from build123d import *

# Parameters (mm, degrees)
SKETCH2_R           = 2.159
BOSS_EXTRUDE3_DEPTH = 3.81
SKETCH1_R           = 38.5318
SKETCH1_R_2         = 35.9918
CUT_EXTRUDE1_DEPTH  = 0.4445
SKETCH4_R           = 25.781
CUT_EXTRUDE2_DEPTH  = 3.81
BOSS_EXTRUDE4_DEPTH = 12.7
BOSS_EXTRUDE5_DEPTH = 6.35
CUT_EXTRUDE3_START  = -3.81
CUT_EXTRUDE3_DEPTH  = 3.81
BOSS_EXTRUDE6_DEPTH = 15.875
CUT_EXTRUDE4_REACH  = 72.276
SKETCH12_R          = 4.2164


with BuildPart() as part:
    # Sketch2 → Boss-Extrude3 (new body)
    with BuildSketch(Plane(origin=(0, 0, 0), x_dir=(1, 0, 0), z_dir=(0, 1, 0))):
        with BuildLine():
            Line((34.29, 46.99), (-34.29, 46.99))
            ThreePointArc((-34.29, 46.99), (-43.270256121, 43.270256121), (-46.99, 34.29))
            Line((-46.99, 34.29), (-46.99, -34.29))
            ThreePointArc((-46.99, -34.29), (-43.270256121, -43.270256121), (-34.29, -46.99))
            Line((-34.29, -46.99), (34.29, -46.99))
            ThreePointArc((34.29, -46.99), (43.270256121, -43.270256121), (46.99, -34.29))
            Line((46.99, -34.29), (46.99, 34.29))
            ThreePointArc((46.99, 34.29), (43.270256121, 43.270256121), (34.29, 46.99))
        make_face()
        with Locations(Location((0, 41.275, 0), (0, 0, 270))):
            Circle(SKETCH2_R, mode=Mode.SUBTRACT)
        with Locations(Location((29.185832393, 29.185832393, 0), (0, 0, 270))):
            Circle(SKETCH2_R, mode=Mode.SUBTRACT)
        with Locations(Location((41.275, 0, 0), (0, 0, 270))):
            Circle(SKETCH2_R, mode=Mode.SUBTRACT)
        with Locations(Location((29.185832393, -29.185832393, 0), (0, 0, 270))):
            Circle(SKETCH2_R, mode=Mode.SUBTRACT)
        with Locations(Location((0, -41.275, 0), (0, 0, 270))):
            Circle(SKETCH2_R, mode=Mode.SUBTRACT)
        with Locations(Location((-29.185832393, -29.185832393, 0), (0, 0, 270))):
            Circle(SKETCH2_R, mode=Mode.SUBTRACT)
        with Locations(Location((-41.275, 0, 0), (0, 0, 270))):
            Circle(SKETCH2_R, mode=Mode.SUBTRACT)
        with Locations(Location((-29.185832393, 29.185832393, 0), (0, 0, 270))):
            Circle(SKETCH2_R, mode=Mode.SUBTRACT)
    extrude(amount=-BOSS_EXTRUDE3_DEPTH)

    # Sketch1 → Cut-Extrude1 (cut)
    with BuildSketch(Plane(origin=(0, 0, 0), x_dir=(1, 0, 0), z_dir=(0, 1, 0))):
        with Locations(Location((0, 0, 0), (0, 0, 270))):
            Circle(SKETCH1_R)
        with Locations(Location((0, 0, 0), (0, 0, 270))):
            Circle(SKETCH1_R_2, mode=Mode.SUBTRACT)
    extrude(amount=-CUT_EXTRUDE1_DEPTH, mode=Mode.SUBTRACT)

    # Sketch4 → Cut-Extrude2 (cut)
    with BuildSketch(Plane(origin=(0, 0, 0), x_dir=(1, 0, 0), z_dir=(0, 1, 0))):
        with Locations(Location((0, 0, 0), (0, 0, 270))):
            Circle(SKETCH4_R)
    extrude(amount=-CUT_EXTRUDE2_DEPTH, mode=Mode.SUBTRACT)

    # Sketch5 → Boss-Extrude4 (add)
    with BuildSketch(Plane.XZ.offset(3.81)):
        with BuildLine():
            ThreePointArc((-29.083, 16.035), (-25.261329281, 25.261329281), (-16.035, 29.083))
            Line((-16.035, 29.083), (16.035, 29.083))
            ThreePointArc((16.035, 29.083), (25.261329281, 25.261329281), (29.083, 16.035))
            Line((29.083, 16.035), (29.083, -16.035))
            ThreePointArc((29.083, -16.035), (25.261329281, -25.261329281), (16.035, -29.083))
            Line((16.035, -29.083), (-16.035, -29.083))
            ThreePointArc((-16.035, -29.083), (-25.261329281, -25.261329281), (-29.083, -16.035))
            Line((-29.083, -16.035), (-29.083, 16.035))
        make_face()
        with BuildLine():
            Line((-26.035, -16.035), (-26.035, 16.035))
            ThreePointArc((-26.035, 16.035), (-23.106067812, 23.106067812), (-16.035, 26.035))
            Line((-16.035, 26.035), (16.035, 26.035))
            ThreePointArc((16.035, 26.035), (23.106067812, 23.106067812), (26.035, 16.035))
            Line((26.035, 16.035), (26.035, -16.035))
            ThreePointArc((26.035, -16.035), (23.106067812, -23.106067812), (16.035, -26.035))
            Line((16.035, -26.035), (-16.035, -26.035))
            ThreePointArc((-16.035, -26.035), (-23.106067812, -23.106067812), (-26.035, -16.035))
        make_face(mode=Mode.SUBTRACT)
    extrude(amount=BOSS_EXTRUDE4_DEPTH)

    # Sketch6 → Boss-Extrude5 (add)
    with BuildSketch(Plane.XZ.offset(16.51)):
        with BuildLine():
            Line((-29.083, 16.035), (-29.083, -16.035))
            ThreePointArc((-29.083, -16.035), (-25.261329281, -25.261329281), (-16.035, -29.083))
            Line((-16.035, -29.083), (16.035, -29.083))
            ThreePointArc((16.035, -29.083), (25.261329281, -25.261329281), (29.083, -16.035))
            Line((29.083, -16.035), (29.083, 16.035))
            ThreePointArc((29.083, 16.035), (25.261329281, 25.261329281), (16.035, 29.083))
            Line((16.035, 29.083), (-16.035, 29.083))
            ThreePointArc((-16.035, 29.083), (-25.261329281, 25.261329281), (-29.083, 16.035))
        make_face()
    extrude(amount=BOSS_EXTRUDE5_DEPTH)

    # Sketch7 → Cut-Extrude3 (cut)
    with BuildSketch(Plane.XZ.offset(3.81).offset(CUT_EXTRUDE3_START)):
        with BuildLine():
            Line((-46.99, 34.29), (-46.99, 0))
            ThreePointArc((-46.99, 0), (-33.226947648, 33.226947648), (0, 46.99))
            Line((0, 46.99), (-34.29, 46.99))
            ThreePointArc((-34.29, 46.99), (-43.270256121, 43.270256121), (-46.99, 34.29))
        make_face()
        with BuildLine():
            ThreePointArc((0, -46.99), (-33.226947648, -33.226947648), (-46.99, 0))
            Line((-46.99, 0), (-46.99, -34.29))
            ThreePointArc((-46.99, -34.29), (-43.270256121, -43.270256121), (-34.29, -46.99))
            Line((-34.29, -46.99), (0, -46.99))
        make_face()
    extrude(amount=CUT_EXTRUDE3_DEPTH, mode=Mode.SUBTRACT)

    # Sketch8 → Boss-Extrude6 (add, symmetric)
    with BuildSketch(Plane(origin=(0, 0, 0), x_dir=(0, 0, -1), z_dir=(1, 0, 0))):
        Polygon((-29.083, -3.81), (-29.083, -11.43), (-34.163, -3.81), align=None)
    boss_extrude6 = extrude(amount=BOSS_EXTRUDE6_DEPTH, both=True)

    # Mirror1: Boss-Extrude6 across plane
    add(boss_extrude6.mirror(Plane.XY))

    # Sketch12 → Cut-Extrude4 (cut, up to next)
    with BuildSketch(Plane.XZ.offset(22.86), mode=Mode.PRIVATE) as cut_extrude4_sk1:
        with Locations(Location((-16.035, 16.035, 0), (0, 0, 270))):
            Circle(SKETCH12_R)
    cut_extrude4_tool1 = extrude(cut_extrude4_sk1.sketch, amount=-CUT_EXTRUDE4_REACH, mode=Mode.PRIVATE) & part.part
    # Sketch12 → Cut-Extrude4 (cut, up to next)
    with BuildSketch(Plane.XZ.offset(22.86), mode=Mode.PRIVATE) as cut_extrude4_sk2:
        with Locations(Location((16.035, -16.035, 0), (0, 0, 270))):
            Circle(SKETCH12_R)
    cut_extrude4_tool2 = extrude(cut_extrude4_sk2.sketch, amount=-CUT_EXTRUDE4_REACH, mode=Mode.PRIVATE) & part.part
    # Sketch12 → Cut-Extrude4 (cut, up to next)
    with BuildSketch(Plane.XZ.offset(22.86), mode=Mode.PRIVATE) as cut_extrude4_sk3:
        with Locations(Location((0, 0, 0), (0, 0, 270))):
            Circle(SKETCH12_R)
    cut_extrude4_tool3 = extrude(cut_extrude4_sk3.sketch, amount=-CUT_EXTRUDE4_REACH, mode=Mode.PRIVATE) & part.part
    add(cut_extrude4_tool1.solids().sort_by_distance((-16.035, -22.86, 16.035))[0], mode=Mode.SUBTRACT)
    add(cut_extrude4_tool2.solids().sort_by_distance((16.035, -22.86, -16.035))[0], mode=Mode.SUBTRACT)
    add(cut_extrude4_tool3.solids().sort_by_distance((0, -22.86, 0))[0], mode=Mode.SUBTRACT)


solid = part.part
Design review of the part built by this model. Coordinates are the model's own, in mm. A direction names the side the tool comes from. Give positions to 0.01 mm unless a question says otherwise; leave off trailing zeros. Order: outer loops, then holes, each group sorted by start corner. A loop starts at its lowest first (then second) coordinate and runs counter-clockwise, first axis right, second up. Notation, with made-up numbers: (30, 29) - (82, 29) arc R26 cw to (82, 65) - close; hole circle Ø1 at (4.5, 46). An arc over 180 degrees is marked (long way). Use CSV: the item, a comma, the result in double quotes. Start each with the question number.
Q1. Take a section at B-B (y = -8.5). State the section outline as (x, z) points (3 decimals).
Q2. For line 1 (X direction, y = -1, z = 0); line 2 (X direction, y = -0.15, z = 0); line 3 (X direction, y = -21.25, z = 0), list the stretches that pass through material, from the lowest coordinate up.
Q3. Draft analysis for pull direction Y (two halves, no side actions). For faces 4 (the face through (0, -22.86, 7)), 5 (the face through (23.18, -10.07, -23.03)), 6 (the face through (43.416, -1.878, -0.281)), 7 (the face through (-23.18, -10.07, 23.03)), state which applies: pulls with the +Y half, pulls with the -Y half, needs draft (parallel to the pull), parting line crosses it, or undercut.
Q4. Take a section at D-D (z = -24). State the section outline as (x, y) points, and give its area (3 significant figures).
Q5. For P1, Ø10, axis at x = 5, y = -16, coming from the -Z side; P2, Ø10, axis at x = -4.5, y = -12, coming from the +Z side; P3, Ø5.5, axis at x = 1, y = -15.5, coming from the -Z side, all flat-tipped, find the tip position at first contact; note any pin that passes through.
Q6. Take a section at A-A (y = -20.5). State the section outline as (x, z) points (3 decimals), and give its area (3 significant figures).
Q7. Take a section at C-C (y = -2.25). Count the separate pieces of the cut face and the enclosed holes in it, and give its area (3 significant figures).
Q8. Machinability: for faces 1 (the face through (25.16, -13.2, -25.36)), 2 (the face through (-15.875, -7, -31)), 3 (the face through (15.875, -7, 31)), which of the approach directions +Z, -Z, +X, -X, +Y, -Y give a long, thin tool a straight path to every point of the face, cutting with its end or side? Answer none if there is none.
Calculated:
1,outline,"(-29.083, -16.035) arc R13.048 ccw to (-16.035, -29.083) - (-15.875, -29.083) - (-15.875, -31.036) - (15.875, -31.036) - (15.875, -29.083) - (16.035, -29.083) arc R13.048 ccw to (29.083, -16.035) - (29.083, 16.035) arc R13.048 ccw to (16.035, 29.083) - (15.875, 29.083) - (15.875, 31.036) - (-15.875, 31.036) - (-15.875, 29.083) - (-16.035, 29.083) arc R13.048 ccw to (-29.083, 16.035) - close; hole (-26.035, -16.035) arc R10 ccw to (-16.035, -26.035) - (16.035, -26.035) arc R10 ccw to (26.035, -16.035) - (26.035, 16.035) arc R10 ccw to (16.035, 26.035) - (-16.035, 26.035) arc R10 ccw to (-26.035, 16.035) - close"
2,line 1,"x = -46.99 to -43.43, -39.12 to -25.78, 25.78 to 39.12, 43.43 to 46.99"
2,line 2,"x = -46.99 to -43.43, -39.12 to -38.53, -35.99 to -25.78, 25.78 to 35.99, 38.53 to 39.12, 43.43 to 46.99"
2,line 3,"x = -29.08 to -4.22, 4.22 to 29.08"
3,face 4,"pulls with the -Y half"
3,face 5,"undercut"
3,face 6,"needs draft"
3,face 7,"undercut"
4,outline,"(-40.4, -3.81) - (-26.37, -3.81) - (-26.37, -22.86) - (26.37, -22.86) - (26.37, -3.81) - (46.99, -3.81) - (46.99, 0) - (30.14, 0) - (30.14, -0.44) - (26.82, -0.44) - (26.82, 0) - (9.42, 0) - (9.42, -3.81) - (22.08, -3.81) - (22.08, -16.51) - (-22.08, -16.51) - (-22.08, -3.81) - (-9.42, -3.81) - (-9.42, 0) - (-26.82, 0) - (-26.82, -0.44) - (-30.14, -0.44) - (-30.14, 0) - (-40.4, 0) - close"
4,area,"702 mm²"
5,P1,"stops at z = -29.37"
5,P2,"stops at z = 32.04"
5,P3,"stops at z = -29.08"
6,outline,"(-29.083, -16.035) arc R13.048 ccw to (-16.035, -29.083) - (16.035, -29.083) arc R13.048 ccw to (29.083, -16.035) - (29.083, 16.035) arc R13.048 ccw to (16.035, 29.083) - (-16.035, 29.083) arc R13.048 ccw to (-29.083, 16.035) - close; hole circle Ø8.433 at (-16.035, 16.035); hole circle Ø8.433 at (0, 0); hole circle Ø8.433 at (16.035, -16.035)"
6,area,"3,070 mm²"
7,separate pieces,"1"
7,enclosed holes,"9"
7,area,"5,610 mm²"
8,face 1,"-Z, +X, -Y"
8,face 2,"-Z, -X, -Y"
8,face 3,"+Z, +X, -Y"
